```python
from build123d import *

# Parameters (mm, degrees)
BOSS_EXTRUDE1_START   = -2.2098
BOSS_EXTRUDE1_DEPTH   = 3.0099
BOSS_EXTRUDE1_2_DEPTH = 2.2098
BOSS_EXTRUDE2_START   = 0.8001
BOSS_EXTRUDE2_DEPTH   = 0.8001
SKETCH3_W             = 1.27
SKETCH3_H             = 2.2098
BOSS_EXTRUDE3_DEPTH   = 0.907414746
SKETCH4_W             = 0.3048
SKETCH4_H             = 3.81
BOSS_EXTRUDE4_DEPTH   = 0.693040986
SKETCH5_W             = 7.6073
SKETCH5_H             = 5.08
BOSS_EXTRUDE5_DEPTH   = 10.6172
SKETCH6_W             = 5.08
SKETCH6_H             = 10.6172
BOSS_EXTRUDE6_DEPTH   = 12.2301
SKETCH7_W             = 19.8374
SKETCH7_H             = 10.6172
BOSS_EXTRUDE7_DEPTH   = 1.27
SKETCH8_W             = 10.8966
SKETCH8_H             = 0.7112
CUT_EXTRUDE1_DEPTH    = 21.314685149
CUT_EXTRUDE2_DEPTH    = 21.314685149
SKETCH10_W            = 0.508
SKETCH10_H            = 3.302
BOSS_EXTRUDE8_DEPTH   = 3.2004
SKETCH11_W            = 0.508
SKETCH11_H            = 3.302
BOSS_EXTRUDE9_DEPTH   = 3.2004
SKETCH12_W            = 0.508
SKETCH12_H            = 3.302
BOSS_EXTRUDE10_DEPTH  = 3.2004
DRAFT1_ANGLE          = 45
SKETCH13_W            = 0.9652
SKETCH13_H            = 3.81
M2_CLEARANCE_HOLE1_D  = 2.413
HOLE1_D               = 1.524
HOLE1_DEPTH           = 4.4323
HOLE2_D               = 1.524
HOLE2_DEPTH           = 0.508
HOLE3_D               = 1.524
HOLE3_DEPTH           = 11.9253
CHAMFER1_SIZE         = 0.127
FILLET1_R             = 0.2032
FILLET2_R             = 0.508
FILLET3_R             = 0.762


with BuildPart() as part:
    # Boss-Extrude1: read off the stored shape, not the designer's step
    # Boss-Extrude1 outline → Boss-Extrude1 (new body)
    with BuildSketch(Plane.XY.offset(1.1049).offset(BOSS_EXTRUDE1_START)):
        with BuildLine():
            ThreePointArc((10.105641195, 13.182599991), (11.032749783, 13.355678114), (11.369702921, 14.236557762))
            Line((11.369702921, 14.236557762), (11.6713, 14.280628634))
            ThreePointArc((11.6713, 14.280628634), (9.96678948, 15.2854128), (9.349347434, 13.405595614))
            Line((9.349347434, 13.405595614), (-7.1247, 11.583182333))
            Line((-7.1247, 11.583182333), (-7.1247, 11.310240986))
            Line((-7.1247, 11.310240986), (-6.8199, 11.310240986))
            Line((-6.8199, 11.310240986), (10.105641195, 13.182599991))
        make_face()
    extrude(amount=BOSS_EXTRUDE1_DEPTH)

    # Boss-Extrude1 2 outline → Boss-Extrude1 2 (add)
    with BuildSketch(Plane.XY.offset(1.1049).offset(BOSS_EXTRUDE1_START)):
        with BuildLine():
            ThreePointArc((-2.3114, 11.524614746), (-2.580781823, 11.679434254), (-2.884355928, 11.745603808))
            Line((-2.884355928, 11.745603808), (-3.228598394, 11.707522575))
            ThreePointArc((-3.228598394, 11.707522575), (-3.414029171, 11.633486118), (-3.5814, 11.524614746))
            Line((-3.5814, 11.524614746), (-2.3114, 11.524614746))
        make_face()
    extrude(amount=BOSS_EXTRUDE1_2_DEPTH)

    # Sketch2 → Boss-Extrude2 (add)
    with BuildSketch(Plane(origin=(0, 0, -1.1049), x_dir=(-1, 0, 0), z_dir=(0, 0, -1)).offset(BOSS_EXTRUDE2_START)):
        with BuildLine():
            Line((6.8199, 11.310240986), (-10.105641195, 13.182599991))
            ThreePointArc((-10.105641195, 13.182599991), (-11.032749783, 13.355678114), (-11.369702921, 14.236557762))
            Line((-11.369702921, 14.236557762), (-11.6713, 14.280628634))
            ThreePointArc((-11.6713, 14.280628634), (-9.96678948, 15.2854128), (-9.349347434, 13.405595614))
            Line((-9.349347434, 13.405595614), (7.1247, 11.583182333))
            Line((7.1247, 11.583182333), (7.1247, 11.310240986))
            Line((7.1247, 11.310240986), (6.8199, 11.310240986))
        make_face()
    extrude(amount=-BOSS_EXTRUDE2_DEPTH)

    # Sketch3 → Boss-Extrude3 (add)
    with BuildSketch(Plane.XZ.offset(-11.524614746)):
        with Locations((-2.9464, 0)):
            Rectangle(SKETCH3_W, SKETCH3_H)
    extrude(amount=BOSS_EXTRUDE3_DEPTH)

    # Sketch4 → Boss-Extrude4 (add)
    with BuildSketch(Plane.XZ.offset(-11.310240986)):
        with Locations((-6.9723, 0)):
            Rectangle(SKETCH4_W, SKETCH4_H)
    extrude(amount=BOSS_EXTRUDE4_DEPTH)

    # Sketch5 → Boss-Extrude5 (add)
    with BuildSketch(Plane.XZ.offset(-10.6172)):
        with Locations((-6.11505, 0.635)):
            Rectangle(SKETCH5_W, SKETCH5_H)
    extrude(amount=BOSS_EXTRUDE5_DEPTH)

    # Sketch6 → Boss-Extrude6 (add)
    with BuildSketch(Plane(origin=(-2.3114, 0, 0), x_dir=(0, 0, -1), z_dir=(1, 0, 0))):
        with Locations((-0.635, 5.3086)):
            Rectangle(SKETCH6_W, SKETCH6_H)
    extrude(amount=BOSS_EXTRUDE6_DEPTH)

    # Sketch7 → Boss-Extrude7 (add)
    with BuildSketch(Plane(origin=(0, 0, -1.905), x_dir=(-1, 0, 0), z_dir=(0, 0, -1))):
        with Locations((0, 5.3086)):
            Rectangle(SKETCH7_W, SKETCH7_H)
    extrude(amount=BOSS_EXTRUDE7_DEPTH)

    # Sketch8 → Cut-Extrude1 (cut, through all)
    with BuildSketch(Plane(origin=(0, 0, -3.175), x_dir=(-1, 0, 0), z_dir=(0, 0, -1))):
        with Locations((-4.4704, 10.2616)):
            Rectangle(SKETCH8_W, SKETCH8_H)
    extrude(amount=-CUT_EXTRUDE1_DEPTH, mode=Mode.SUBTRACT)

    # Sketch9 → Cut-Extrude2 (cut, through all)
    with BuildSketch(Plane(origin=(0, 0, -3.175), x_dir=(-1, 0, 0), z_dir=(0, 0, -1))):
        with BuildLine():
            Line((4.9149, 4.064), (4.6609, 4.064))
            ThreePointArc((4.6609, 4.064), (3.4544, 2.8575), (4.6609, 1.651))
            Line((4.6609, 1.651), (4.9149, 1.651))
            ThreePointArc((4.9149, 1.651), (6.1214, 2.8575), (4.9149, 4.064))
        make_face()
    extrude(amount=-CUT_EXTRUDE2_DEPTH, mode=Mode.SUBTRACT)

    # Sketch10 → Boss-Extrude8 (add)
    with BuildSketch(Plane.XZ):
        Rectangle(SKETCH10_W, SKETCH10_H)
    extrude(amount=BOSS_EXTRUDE8_DEPTH)

    # Sketch11 → Boss-Extrude9 (add)
    with BuildSketch(Plane.XZ):
        with Locations((-7.493, 0)):
            Rectangle(SKETCH11_W, SKETCH11_H)
    extrude(amount=BOSS_EXTRUDE9_DEPTH)

    # Sketch12 → Boss-Extrude10 (add)
    with BuildSketch(Plane.XZ):
        with Locations((7.493, 0)):
            Rectangle(SKETCH12_W, SKETCH12_H)
    extrude(amount=BOSS_EXTRUDE10_DEPTH)

    # Draft1
    draft1_faces = [part.faces().sort_by_distance(p)[0] for p in [
        (-0.9779, 10.2616, 0),
    ]]
    draft(draft1_faces, Plane(origin=(0, 10.6172, 0), x_dir=(1, 0, 0), z_dir=(0, 1, 0)), DRAFT1_ANGLE)

    # Sketch13 → Cut-Revolve1 (revolve, cut)
    with BuildSketch(Plane.XZ.offset(-14.097)):
        with Locations((10.897245503, 0)):
            Rectangle(SKETCH13_W, SKETCH13_H)
    revolve(axis=Axis((10.414645503, 14.097, 1.905), (0, 0, -1)), mode=Mode.SUBTRACT)

    # M2 Clearance Hole1 (through all)
    with Locations(Plane.XY.offset(3.175)):
        with Locations((4.7117, 2.8575)):
            Hole(M2_CLEARANCE_HOLE1_D / 2)

    # Hole1
    with Locations(Plane.ZY.offset(-7.239)):
        with Locations((0, -1.6764)):
            Hole(HOLE1_D / 2, depth=HOLE1_DEPTH)

    # Hole2
    with Locations(Plane.ZY.offset(7.747)):
        with Locations((0, -1.6764)):
            Hole(HOLE2_D / 2, depth=HOLE2_DEPTH)

    # Hole3
    with Locations(Plane.ZY.offset(0.254)):
        with Locations((0, -1.6764)):
            Hole(HOLE3_D / 2, depth=HOLE3_DEPTH)

    # Chamfer1
    chamfer1_edges = [part.edges().sort_by_distance(p)[0] for p in [
        (0, -3.2004, -1.651),
        (0, -3.2004, 1.651),
        (-7.493, -3.2004, -1.651),
        (-7.493, -3.2004, 1.651),
        (7.493, -3.2004, -1.651),
        (7.493, -3.2004, 1.651),
    ]]
    chamfer(chamfer1_edges, length=CHAMFER1_SIZE)

    # Fillet1
    fillet1_edges = [part.edges().sort_by_distance(p)[0] for p in [
        (-6.8199, 11.310240986, 0.40005),
    ]]
    fillet(fillet1_edges, radius=FILLET1_R)

    # Fillet2
    fillet2_edges = [part.edges().sort_by_distance(p)[0] for p in [
        (-7.1247, 11.583182333, 0.40005),
        (9.349347434, 13.405595614, 0.40005),
    ]]
    fillet(fillet2_edges, radius=FILLET2_R)

    # Fillet3
    fillet3_edges = [part.edges().sort_by_distance(p)[0] for p in [
        (10.105641195, 13.182599991, 0.40005),
        (-9.9187, 10.6172, 0),
        (9.9187, 9.906, 0),
    ]]
    fillet(fillet3_edges, radius=FILLET3_R)


solid = part.part
```
The model under review builds one solid part; all positions refer to its coordinate system, in mm. A direction names the side the tool comes from. Coordinates: 2 decimals unless noted, no trailing zeros. Write each loop counter-clockwise with the first axis right and the second up, starting at its lowest first coordinate (ties: lowest second). Pieces come first, ordered by that corner, then holes. Notation, with made-up numbers: (-4, 27.5) -> (26, 27.5) arc R27 cw to (26, 50.5) -> close; hole circle Ø4 at (53, 87). An arc over 180 degrees is marked (long way). One line per item, written item: value. Start each with the question number.
Q1. Add section D-D, the plane x = -4. Give the boundary of the cut face in (y, z) (3 decimals), then the cut area to 3 significant figures.
Q2. The part is to be moulded in two halves that separate along Y. For faces 1 (the face through (1.127, 12.496, -0.027)), 2 (the face through (7.747, -2, -1)), 3 (the face through (0.97, 12.17, -0.03)), say which applies: +Y half, -Y half, draft (parallel to the pull), parting line (faces both ways), or undercut.
Q3. Add section C-C, the plane x = -1.25. Give the boundary of the cut face in (y, z) (3 decimals), then the cut area to 3 significant figures.
Q4. For faces 4 (the face through (-3, 11, 1.105)), 5 (the face through (7.239, -2, -1)), 6 (the face through (9.33, 13.35, 0.03)), 7 (the face through (-3.455, 2.884, -0.044)), 8 (the face through (-7.747, -2, -1)), list the 3-axis set-ups (+Z, -Z, +X, -X, +Y, -Y) from which the entire face can be reached by the end or side of a thin tool; tool diameter is ignored.
Q5. Add section B-B, the plane z = 2.25. Give the boundary of the cut face in (x, y).
Q6. Clearance check with flat-ended pins moving along their axes: P1, Ø0.6, axis at x = -3, y = 11, coming from the +Z side; P2, Ø2.5, axis at y = -1.68, z = 0, coming from the -X side; P3, Ø3, axis at x = 2.5, y = 11.5, coming from the -Z side (3 decimals); P4, Ø6, axis at x = 5, y = -0.5, coming from the +Z side (3 decimals). State where each tip first meets the part, or that it passes through.
Q7. Add section A-A, the plane y = 2.25. Give the boundary of the cut face in (x, z) (1 decimal), then the cut area to 3 significant figures.
Q8. To check wall thickness, follow probe 1 along X at (y, z) = (-1, 0.5); probe 2 along Y at (x, z) = (-4.75, -1.5); probe 3 along Y at (x, z) = (7.55, 0). State the ranges of each line that lie inside material, in increasing order.
Response:
1. outline: (0, -3.175) -> (1.848, -3.175) -> (1.848, 3.175) -> (0, 3.175) -> close; (3.867, -3.175) -> (10.617, -3.175) -> (10.617, 3.175) -> (3.867, 3.175) -> close; (11.622, -1.905) -> (11.929, -1.905) -> (11.929, 1.905) -> (11.622, 1.905) -> close
1. area: 55.8 mm²
2. face 1: +Y half
2. face 2: draft
2. face 3: undercut
3. outline: (0, -3.175) -> (10.617, -3.175) -> (10.617, 3.175) -> (0, 3.175) -> close; (11.926, -1.905) -> (12.233, -1.905) -> (12.233, 1.905) -> (11.926, 1.905) -> close
3. area: 68.6 mm²
4. face 4: +Z, +X
4. face 5: +Z, -Z, -Y
4. face 6: +Z, -Z, +X
4. face 7: +Z, -Z
4. face 8: +Z, -Z, -X, -Y
5. outline: (-9.92, 0) -> (9.92, 0) -> (9.92, 9.14) arc R0.76 ccw to (9.16, 9.91) -> (-0.27, 9.91) -> (-0.98, 10.62) -> (-9.16, 10.62) arc R0.76 ccw to (-9.92, 9.86) -> close; hole (-4.91, 1.65) -> (-4.66, 1.65) arc R1.21 ccw to (-4.66, 4.06) -> (-4.91, 4.06) arc R1.21 ccw to start; hole circle Ø2.41 at (4.71, 2.86)
6. P1: z = 1.1
6. P2: x = -7.75
6. P3: z = -1.905
6. P4: z = 3.175
7. outline: (-9.9, -3.2) -> (-6, -3.2) -> (-6, 3.2) -> (-9.9, 3.2) -> close; (-3.6, -3.2) -> (3.7, -3.2) -> (3.7, 3.2) -> (-3.6, 3.2) -> close; (5.8, -3.2) -> (9.9, -3.2) -> (9.9, 3.2) -> (5.8, 3.2) -> close
7. area: 97.9 mm²
8. probe 1: -7.75 to -7.24, -0.25 to 0.25, 7.24 to 7.75
8. probe 2: 0 to 1.65, 4.06 to 10.62, 11.54 to 11.85
8. probe 3: -3.2 to -2.44, -0.91 to 9.91, 12.9 to 13.21
